Build history of the part. All positions in model axes, mm. Round coordinates to 2 decimals unless told otherwise and drop trailing zeros. Order: outer loops, then holes, each group sorted by start corner. A loop starts at its lowest first (then second) coordinate and runs counter-clockwise, first axis right, second up. Notation, with made-up numbers: (78.25, 83.25) -> (108.25, 83.25) arc R7 cw to (108.25, 92.25) -> close; hole circle Ø1 at (19, -4). An arc over 180 degrees is marked (long way). Write item = value, one per line.
from build123d import *

# Parameters (mm, degrees)
SKETCH1_W           = 500
SKETCH1_H           = 168.89
BOSS_EXTRUDE1_DEPTH = 12
SKETCH2_W           = 166.666666666
SKETCH2_H           = 12
CUT_EXTRUDE1_DEPTH  = 528.889981057
SKETCH4_W           = 12
SKETCH4_H           = 56.296666667
CUT_EXTRUDE3_DEPTH  = 528.889981057
CUT_EXTRUDE4_DEPTH  = 528.889981057
LPATTERN1_COUNT     = 3
LPATTERN1_PITCH     = 50
SCALE1_SCALE        = 0.5


with BuildPart() as part:
    # Sketch1 → Boss-Extrude1 (new body)
    with BuildSketch(Plane(origin=(0, 0, 0), x_dir=(1, 0, 0), z_dir=(0, 1, 0))):
        with Locations((250, 84.445)):
            Rectangle(SKETCH1_W, SKETCH1_H)
    extrude(amount=BOSS_EXTRUDE1_DEPTH)

    # Sketch2 → Cut-Extrude1 (cut, through all)
    with BuildSketch(Plane(origin=(0, 12, 0), x_dir=(1, 0, 0), z_dir=(0, 1, 0))):
        with Locations((250, 6)):
            Rectangle(SKETCH2_W, SKETCH2_H)
    extrude(amount=-CUT_EXTRUDE1_DEPTH, mode=Mode.SUBTRACT)

    # Sketch4 → Cut-Extrude3 (cut, through all)
    with BuildSketch(Plane(origin=(0, 12, 0), x_dir=(1, 0, 0), z_dir=(0, 1, 0))):
        with Locations((6, 140.741666667)):
            Rectangle(SKETCH4_W, SKETCH4_H)
        with Locations((6, 28.148333334)):
            Rectangle(SKETCH4_W, SKETCH4_H)
        with Locations((494, 28.148333334)):
            Rectangle(SKETCH4_W, SKETCH4_H)
        with Locations((494, 140.741666667)):
            Rectangle(SKETCH4_W, SKETCH4_H)
    extrude(amount=-CUT_EXTRUDE3_DEPTH, mode=Mode.SUBTRACT)

    # Sketch5 → Cut-Extrude4 (cut, through all)
    with BuildSketch(Plane(origin=(0, 12, 0), x_dir=(1, 0, 0), z_dir=(0, 1, 0))):
        with BuildLine():
            Line((55.5, 153.449523313), (444.5, 153.449523313))
            ThreePointArc((444.5, 153.449523313), (448.389087297, 151.838610609), (450, 147.949523313))
            Line((450, 147.949523313), (450, 146.949523313))
            ThreePointArc((450, 146.949523313), (448.389087297, 143.060436016), (444.5, 141.449523313))
            Line((444.5, 141.449523313), (55.5, 141.449523313))
            ThreePointArc((55.5, 141.449523313), (51.610912703, 143.060436016), (50, 146.949523313))
            Line((50, 146.949523313), (50, 147.949523313))
            ThreePointArc((50, 147.949523313), (51.610912703, 151.838610609), (55.5, 153.449523313))
        make_face()
    cut_extrude4 = extrude(amount=-CUT_EXTRUDE4_DEPTH, mode=Mode.SUBTRACT)

    # LPattern1: Cut-Extrude4 ×3
    with Locations(*[(0, 0, i * LPATTERN1_PITCH) for i in range(1, LPATTERN1_COUNT)]):
        add(cut_extrude4, mode=Mode.SUBTRACT)


with BuildPart() as part_1:
    # Scale1: scaled about (250, 6, -83.99618036)
    add(part.part.scale(SCALE1_SCALE).moved(Location((125, 3, -41.99809018))))


solid = part_1.part
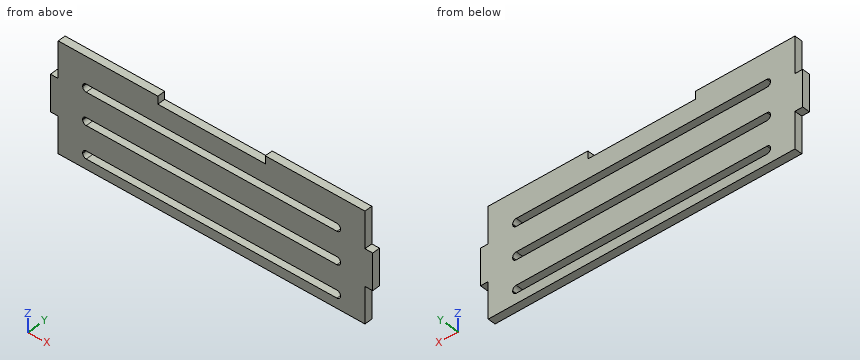
Q1. Cut at D-D, the plane z = -107.5. List the corners of the cut face in (x, y), and give its area (3 significant figures).
Check values:
outline = (131, 3) -> (369, 3) -> (369, 9) -> (131, 9) -> close
area = 1,430 mm²
Q2. Cut at A-A, the plane x = 183. List the corners of the cut face in (y, z).
Check values:
outline = (3, -126.44) -> (9, -126.44) -> (9, -118.72) -> (3, -118.72) -> close; (3, -112.72) -> (9, -112.72) -> (9, -93.72) -> (3, -93.72) -> close; (3, -87.72) -> (9, -87.72) -> (9, -68.72) -> (3, -68.72) -> close; (3, -62.72) -> (9, -62.72) -> (9, -42) -> (3, -42) -> close
Q3. Cut at C-C, the plane x = 250. List the corners of the cut face in (y, z), and give its area (3 significant figures).
Check values:
outline = (3, -126.44) -> (9, -126.44) -> (9, -118.72) -> (3, -118.72) -> close; (3, -112.72) -> (9, -112.72) -> (9, -93.72) -> (3, -93.72) -> close; (3, -87.72) -> (9, -87.72) -> (9, -68.72) -> (3, -68.72) -> close; (3, -62.72) -> (9, -62.72) -> (9, -48) -> (3, -48) -> close
area = 363 mm²
Q4. Probe probe 1 along Z at (x, y) = (324, 5.4); probe 2 along Z at (x, y) = (271.5, 7.15); probe 3 along X at (y, z) = (8.75, -98.5). List the from-to ranges inside material, lowest first.
Check values:
probe_1 = -126.44 to -118.72, -112.72 to -93.72, -87.72 to -68.72, -62.72 to -42
probe_2 = -126.44 to -118.72, -112.72 to -93.72, -87.72 to -68.72, -62.72 to -48
probe_3 = 131 to 369
Q5. Cut at B-B, the plane y = 7.5. Give the number of separate pieces and of enclosed holes in the cut face, and give its area (3 significant figures).
Check values:
separate_pieces = 1
enclosed_holes = 3
area = 16,400 mm²
Q6. Flat gauge pins, fed straight in: pin 1 (1.5 mm diameter, centred on y = 6, z = -111.5, fed in from +X); pin 2 (3 mm diameter, centred on y = 7.5, z = -43.5, fed in from -X); pin 3 (3 mm diameter, centred on x = 371.5, y = 4.5, fed in from -Z). Where does each tip first touch, or does it go through?
Check values:
pin_1 = 369
pin_2 = 131
pin_3 = -98.29
